```python
from build123d import *

# Parameters (mm, degrees)
F1_DEPTH = 60
F2_R     = 29.99999
F3_R     = 15
F4_DEPTH = 10
F5_R     = 5
F6_DEPTH = 10
F7_W     = 46
F7_H     = 15
F8_DEPTH = 10
F9_R     = 5
F10_R    = 5


# Not quite as in the source:
# - a fillet or chamfer is up to 0.001 mm smaller than in the source, because OpenCascade refuses the exact size


with BuildPart() as f1:
    # F0 (on Front) → F1 (new body)
    with BuildSketch(Plane.XZ):
        Polygon((80, 0), (0, 0), (0, -10), (77.3205080757, -10), (126.9615242271, -38.6602540378), (131.9615242271, -30), align=None)
    extrude(amount=F1_DEPTH)

    # F2 (radius 30 in the source; OpenCascade refuses exactly that, so slightly less here)
    f2_edges = [f1.edges().sort_by_distance(p)[0] for p in [
        (129.461524, 0, -34.330127),
        (129.461524, -60, -34.330127),
    ]]
    fillet(f2_edges, radius=F2_R)

    # F3 (on face) → F4 (cut, through all)
    with BuildSketch(Plane(origin=(20, 0, 34.6410161514), x_dir=(0.8660254038, 0, -0.5), z_dir=(0.5, 0, 0.8660254038))):
        with Locations((99.2820323028, -30)):
            Circle(F3_R)
    extrude(amount=-F4_DEPTH, mode=Mode.SUBTRACT)

    # F5 (on face) → F6 (cut, through all)
    with BuildSketch(Plane.XY):
        with Locations((12, -13)):
            Circle(F5_R)
        with Locations((12, -48)):
            Circle(F5_R)
        with Locations((62, -48)):
            Circle(F5_R)
        with Locations((62, -13)):
            Circle(F5_R)
    extrude(amount=-F6_DEPTH, mode=Mode.SUBTRACT)

    # F7 (on face) → F8 (cut, through all)
    with BuildSketch(Plane.XY):
        with Locations((40, -30)):
            Rectangle(F7_W, F7_H)
    extrude(amount=-F8_DEPTH, mode=Mode.SUBTRACT)

    # F9
    f9_edges = [f1.edges().sort_by_distance(p)[0] for p in [
        (17, -22.5, -5),
    ]]
    fillet(f9_edges, radius=F9_R)

    # F10
    f10_edges = [f1.edges().sort_by_distance(p)[0] for p in [
        (63, -22.5, -5),
        (63, -37.5, -5),
        (17, -37.5, -5),
    ]]
    fillet(f10_edges, radius=F10_R)


solid = f1.part
```
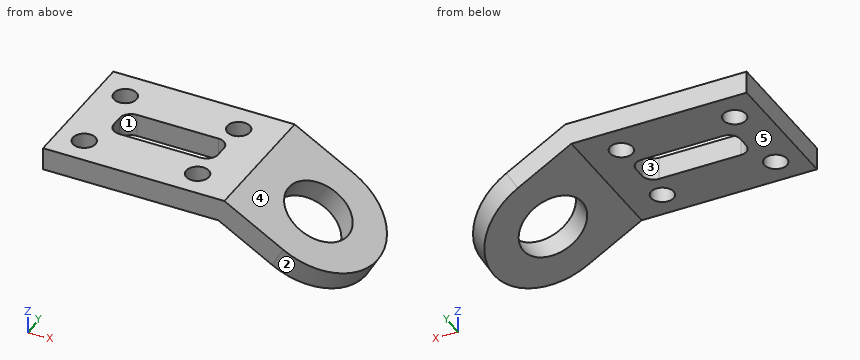
Input: part model. Units: mm. Frame: model coordinates. Face numbers are marked on the shaded views. A direction names the side the tool comes from. Give positions to 0.01 mm unless a question says otherwise; leave off trailing zeros. Order: outer loops, then holes, each group sorted by start corner. A loop starts at its lowest first (then second) coordinate and runs counter-clockwise, first axis right, second up. Notation, with made-up numbers: (20, 26) - (39, 26) arc R33 ccw to (39, 54) - close; hole circle Ø11 at (57.5, 83). An arc over 180 degrees is marked (long way). Use a Markdown table: item, result.
(1) Section query B-B (y = -50.5). Output: boundary loops of the cut face in (x, z).
Computed values:
| item | result |
|---|---|
| outline | (0, -10) - (7.67, -10) - (7.67, 0) - (0, 0) - close; (16.33, -10) - (57.67, -10) - (57.67, 0) - (16.33, 0) - close; (66.33, -10) - (77.32, -10) - (119.95, -34.61) - (124.95, -25.95) - (80, 0) - (66.33, 0) - close |
(2) Section query A-A (x = 54). Output: boundary loops of the cut face in (y, z), then the cut area to 3 significant figures.
Computed values:
| item | result |
|---|---|
| outline | (-60, -10) - (-37.5, -10) - (-37.5, 0) - (-60, 0) - close; (-22.5, -10) - (0, -10) - (0, 0) - (-22.5, 0) - close |
| area | 450 mm2 |
(3) Pin query (flat end, axial travel): pin 1 (4 mm diameter, centred on x = 33.5, y = -11, fed in from -Z); pin 2 (2.5 mm diameter, centred on y = -31, z = -6, fed in from +X); pin 3 (9 mm diameter, centred on x = 12, y = -48, fed in from -Z); pin 4 (10 mm diameter, centred on y = -44, z = -23.5, fed in from +X). Return the tip coordinate at first contact, or that it passes through.
Computed values:
| item | result |
|---|---|
| pin 1 | stops at z = -10 |
| pin 2 | stops at x = 92.56 |
| pin 3 | passes through |
| pin 4 | stops at x = 129.27 |
(4) Section query C-C (x = 12). Output: boundary loops of the cut face in (y, z).
Computed values:
| item | result |
|---|---|
| outline | (-60, -10) - (-53, -10) - (-53, 0) - (-60, 0) - close; (-43, -10) - (-18, -10) - (-18, 0) - (-43, 0) - close; (-8, -10) - (0, -10) - (0, 0) - (-8, 0) - close |
(5) Section query D-D (z = -5.5). Output: boundary loops of the cut face in (x, y), then the cut area to 3 significant figures.
Computed values:
| item | result |
|---|---|
| outline | (0, -60) - (89.53, -60) - (89.53, 0) - (0, 0) - close; hole circle Ø10 at (12, -48); hole circle Ø10 at (12, -13); hole (17, -32.5) arc R5 ccw to (22, -37.5) - (58, -37.5) arc R5 ccw to (63, -32.5) - (63, -27.5) arc R5 ccw to (58, -22.5) - (22, -22.5) arc R5 ccw to (17, -27.5) - close; hole circle Ø10 at (62, -48); hole circle Ø10 at (62, -13) |
| area | 4,390 mm2 |
(6) Access query for the marked faces 1 and 2. Directions: +Z, -Z, +X, -X, +Y, -Y. A direction counts if a zero-diameter tool reaches every point of the face in a straight line with its end or side. Return the directions, or none.
Computed values:
| item | result |
|---|---|
| face 1 | +Z, -Z |
| face 2 | -Z, +X, -Y |
(7) Draft query along X for the marked faces 3, 4 and 5. Return one class per face: released by +X, released by -X, zero draft, split by the parting line, or undercut.
Computed values:
| item | result |
|---|---|
| face 3 | undercut |
| face 4 | released by +X |
| face 5 | zero draft |
(8) Line query: line 1 (Y direction, x = 12, z = -1.75); line 2 (Y direction, x = 62, z = -3); line 3 (Z direction, x = 64, y = -18). Output: solid intervals per line, ascending. Write a range as from..to.
Computed values:
| item | result |
|---|---|
| line 1 | y = -60..-53, -43..-18, -8..0 |
| line 2 | y = -60..-53, -43..-35.5, -24.5..-18, -8..0 |
| line 3 | z = -10..0 |
